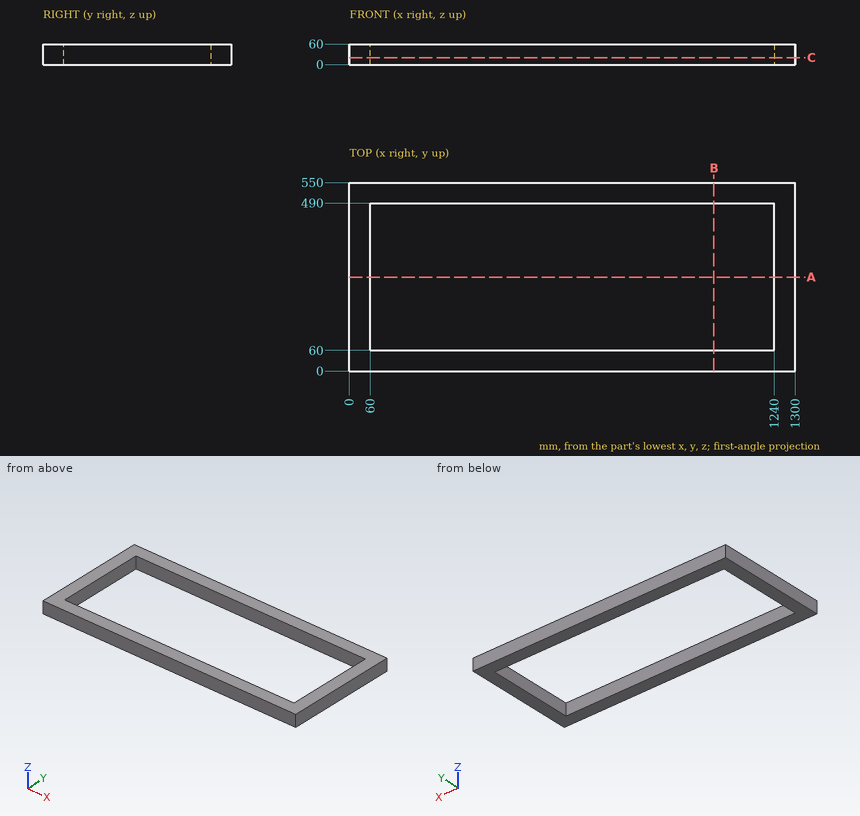
Drawing for the job (mm, zero at the part's lowest x, y, z). Give positions to 0.01 mm unless a question says otherwise; leave off trailing zeros. Loops run counter-clockwise (first coordinate to the right, second up) from the corner with the lowest first, then second, coordinate; pieces in that order, holes last.
(1) Drill centre lines: line 1 along Y through (x, z) = (1048, 48); line 2 along X through (y, z) = (191, 10). Where is each one in solid material? Low to high.
Return value:
line 1: y = 0 to 60, 490 to 550
line 2: x = 0 to 60, 1240 to 1300
(2) Band-saw the part on B-B (x = 1063.5). Write the cut outline in (y, z), and give its area (3 significant figures).
Return value:
outline: (0, 0) - (60, 0) - (60, 60) - (0, 60) - close; (490, 0) - (550, 0) - (550, 60) - (490, 60) - close
area: 7,200 mm2
(3) Band-saw the part on A-A (y = 274). Write the cut outline in (x, z), and give its area (3 significant figures).
Return value:
outline: (0, 0) - (60, 0) - (60, 60) - (0, 60) - close; (1240, 0) - (1300, 0) - (1300, 60) - (1240, 60) - close
area: 7,200 mm2
(4) Band-saw the part on C-C (z = 20). Write the cut outline in (x, y).
Return value:
outline: (0, 0) - (1300, 0) - (1300, 550) - (0, 550) - close; hole (60, 60) - (1240, 60) - (1240, 490) - (60, 490) - close
